Autodesk Inventor part; units mm, degrees
ref_plane "YZ Plane" through (0, 0, 0) normal (1, 0, 0) x (0, 1, 0)
ref_plane "XZ Plane" through (0, 0, 0) normal (0, 1, 0) x (-1, 0, 0)
ref_plane "XY Plane" through (0, 0, 0) normal (0, 0, 1) x (1, 0, 0)
sketch "Base Pattern" plane through (0, 0, 0) normal (0, 1, 0) x (-1, 0, 0)
  line L0 (50, 13.5) -> (-50, 13.5)
  line L1 (-50, 13.5) -> (-50, -13.5)
  line L2 (-50, -13.5) -> (50, -13.5)
  line L3 (50, -13.5) -> (50, 13.5)
  line L4 (50, 13.5) -> (-50, -13.5) construction
  line L5 (-50, 13.5) -> (50, -13.5) construction
  point P0 (0, 0)
  dimension "Length" = 100
  dimension "Base_Width" = 27
sketch "Slot Pattern Set-Out" plane through (0, 0, 0) normal (0, 1, 0) x (-1, 0, 0)
  line L0 (0, -25) -> (0, 25)
  line L1 (9.9, 2.6) -> (-9.9, 2.6)
  line L2 (-9.9, -2.6) -> (9.9, -2.6)
  arc A0 (9.9, -2.6) -> (9.9, 2.6) centre (9.9, 0) ccw
  arc A1 (-9.9, 2.6) -> (-9.9, -2.6) centre (-9.9, 0) ccw
  line L3 (32, 0) -> (-32, 0) construction
  line L4 (9.9, 0) -> (-9.9, 0) construction
  point P0 (0, 0)
  point P1 (0, 0)
  point P2 (0, 0)
  point P3 (0, 0)
  dimension "Slot_Length" = 19.8
  dimension "Slot_Dia" = 5.2
  dimension "Pattern_Length" = 64
extrude "Plate1" add sketch "Base Pattern" along normal blind 1
sketch "Sketch3" plane through (-50, 0, -12.5) normal (0, 0, -1) x (-1, 0, 0)
  line L0 (-100, 0) -> (0, 0)
  line L1 (0, 0) -> (0, 7.5)
  line L2 (0, 7.5) -> (-100, 7.5)
  line L3 (-100, 7.5) -> (-100, 0)
edge flange "Flange Side" height 7.5 angle 90 thickness 1 bend radius 1 thickness toward (0, 0, -1) relief tear relief width 1 relief depth 0.5 corner gap 1 corner form 0 edges at (0, 1, -13.5) (0, 1, 13.5) wall of the first edge with corners at (50, 0, -12.5) (-50, 0, -12.5) (-50, 7.5, -12.5) (50, 7.5, -12.5)
bend "Bend1"
corner "Corner1"
sketch "Sketch4" plane through (-50, 7.5, 13.5) normal (0, 1, 0) x (-1, 0, 0)
  line L0 (-100, 0) -> (0, 0)
  line L1 (0, 0) -> (0, 4)
  line L2 (0, 4) -> (-100, 4)
  line L3 (-100, 4) -> (-100, 0)
edge flange "Flange Nib" height 5 angle 90 thickness 1 bend radius 1 thickness toward (0, 1, 0) relief tear relief width 1 relief depth 0.5 corner gap 1 corner form 0 edges at (0, 7.5, 13.5) (0, 7.5, -13.5) wall of the first edge with corners at (50, 7.5, 13.5) (-50, 7.5, 13.5) (-50, 7.5, 17.5) (50, 7.5, 17.5)
bend "Bend2"
corner "Corner2"
extrude "Slot Cut-Out" cut sketch "Slot Pattern Set-Out" along normal blind 1
pattern_linear "Slot Pattern" count 2 spacing 36 along (1, 0, 0) of "Slot Cut-Out"
mirror "Slot Patern Mirror" about plane through (0, 0, 0) normal (1, 0, 0) of "Slot Cut-Out", "Slot Pattern"
equation "\"Slot_Length\" = Slot_Length_Effective"
equation "\"d28\" = Thickness"
equation "\"d30\" = 0.6 * Slots_Integer"
equation "\"d32\" = Slot_Spacing"
equation "\"d8\" = BendReliefWidth"
equation "\"d9\" = BendReliefDepth"
equation "\"d10\" = MinimumRemnant"
equation "\"d11\" = BendRadius"
equation "\"d12\" = Flange_Height"
equation "\"d14\" = BendRadius"
equation "\"d15\" = CornerReliefSize"
equation "\"d16\" = GapSize"
equation "\"d17\" = JacobiRadiusSize"
equation "\"d18\" = BendReliefWidth"
equation "\"d19\" = BendReliefDepth"
equation "\"d20\" = MinimumRemnant"
equation "\"d21\" = BendRadius"
equation "\"d22\" = Flange_Nib"
equation "\"d24\" = BendRadius"
equation "\"d25\" = CornerReliefSize"
equation "\"d26\" = GapSize"
equation "\"d27\" = JacobiRadiusSize"
equation "\"BendRadius\" = Thickness"
equation "\"BendReliefWidth\" = Thickness"
equation "\"BendReliefDepth\" = 0.5 * Thickness"
equation "\"CornerReliefSize\" = 4 * Thickness"
equation "\"MinimumRemnant\" = 2 * Thickness"
equation "\"TransitionRadius\" = BendRadius"
equation "\"JacobiRadiusSize\" = BendRadius"
equation "\"GapSize\" = Thickness"
equation "\"Flange_Height\" = 7.5"
equation "\"Slot_Spacing\" = 36"
equation "\"Flange_Nib\" = 5"
equation "\"Slot_Length_Tab\" = 25"
equation "\"Slot_Length_Effective\" = Slot_Length_Tab - Slot_Dia"
properties part number "DIN Rail (TS) 35mm Wide v1-01" material "Steel"
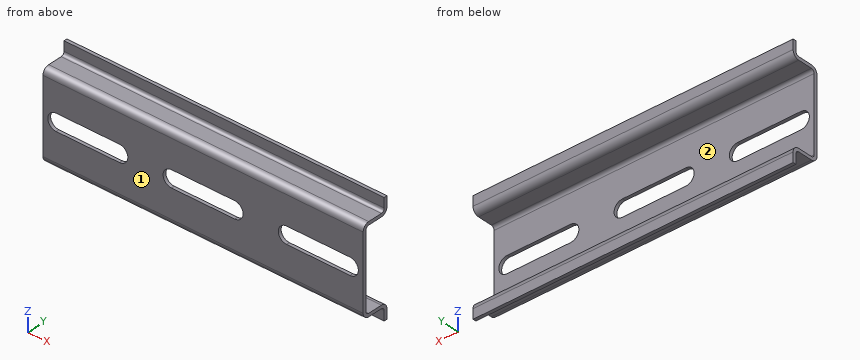
Build history of the part. All positions in model axes, mm. Face numbers are marked on the shaded views. Round coordinates to 2 decimals unless told otherwise and drop trailing zeros. Write each loop counter-clockwise with the first axis right and the second up, starting at its lowest first coordinate (ties: lowest second). Pieces come first, ordered by that corner, then holes. Notation, with made-up numbers: M 12,74.25 L 24,74.25 A22 cw 24,85.25 Z; hole C 43.5,41 d2. An arc over 180 degrees is marked long. Answer as a JSON object with one key per item and string values. Group by question number.
(1) Cut at D-D (x = -22). Give the cut face in (y, z).
(2) Cut at A-A (z = 0). Give the cut face in (x, y).
(3) Flat gauge pins, fed straight in: pin 1 (3 mm diameter, centred on x = -4.5, y = 1, fed in from +Z); pin 2 (0.9 mm diameter, centred on x = 14.5, z = 15.5, fed in from -Y); pin 3 (1.1 mm diameter, centred on x = -2, y = 0.5, fed in from -Z). Where does each tip first touch, or does it go through?
(4) Cut at B-B (x = -39). Give the cut face in (y, z).
(5) Mould opens along Z. For the marked faces 1 and 2 say: pulls with the +Z half, pulls with the -Z half, needs draft (parallel to the pull), parting line crosses it, or undercut.
(6) Drill centre lines: L1, parallel to Z at x = -39, y = 2.75; L2, parallel to Y at x = 1.5, z = 9.5; L3, parallel to Z at x = 13, y = 7. Where is each one in solid material? Low to high.
(7) Cut at C-C (y = 5.5). Give the cut face in (x, z), and give its area (3 significant figures).
Responses:
{
 "1": {"outline": "M 0,-11.5 A2 ccw 2,-13.5 L 6.5,-13.5 A1 cw 7.5,-14.5 L 7.5,-17.5 L 8.5,-17.5 L 8.5,-14.5 A2 ccw 6.5,-12.5 L 2,-12.5 A1 cw 1,-11.5 L 1,11.5 A1 cw 2,12.5 L 6.5,12.5 A2 ccw 8.5,14.5 L 8.5,17.5 L 7.5,17.5 L 7.5,14.5 A1 cw 6.5,13.5 L 2,13.5 A2 ccw 0,11.5 Z"},
 "2": {"outline": "M -50,0 L -48.5,0 L -48.5,1 L -50,1 Z; M -23.5,0 L -12.5,0 L -12.5,1 L -23.5,1 Z; M 12.5,0 L 23.5,0 L 23.5,1 L 12.5,1 Z; M 48.5,0 L 50,0 L 50,1 L 48.5,1 Z"},
 "3": {"pin 1": "stops at z = 13.5", "pin 2": "stops at y = 7.5", "pin 3": "stops at z = -13.26"},
 "4": {"outline": "M 0,-11.5 A2 ccw 2,-13.5 L 6.5,-13.5 A1 cw 7.5,-14.5 L 7.5,-17.5 L 8.5,-17.5 L 8.5,-14.5 A2 ccw 6.5,-12.5 L 2,-12.5 A1 cw 1,-11.5 L 1,-2.6 L 0,-2.6 Z; M 0,2.6 L 1,2.6 L 1,11.5 A1 cw 2,12.5 L 6.5,12.5 A2 ccw 8.5,14.5 L 8.5,17.5 L 7.5,17.5 L 7.5,14.5 A1 cw 6.5,13.5 L 2,13.5 A2 ccw 0,11.5 Z"},
 "5": {"face 1": "needs draft", "face 2": "undercut"},
 "6": {"L1": "z = -13.5 to -12.5, 12.5 to 13.5", "L2": "y = 0 to 1", "L3": "z = -13.63 to -12.56, 12.56 to 13.63"},
 "7": {"outline": "M -50,-13.5 L 50,-13.5 L 50,-12.5 L -50,-12.5 Z; M -50,12.5 L 50,12.5 L 50,13.5 L -50,13.5 Z", "area": "200 mm2"}
}
